Drawing for the job (mm, zero at the part's lowest x, y, z). A direction names the side the tool comes from. Coordinates: 2 decimals unless noted, no trailing zeros. Write each loop counter-clockwise with the first axis right and the second up, starting at its lowest first coordinate (ties: lowest second). Pieces come first, ordered by that corner, then holes.
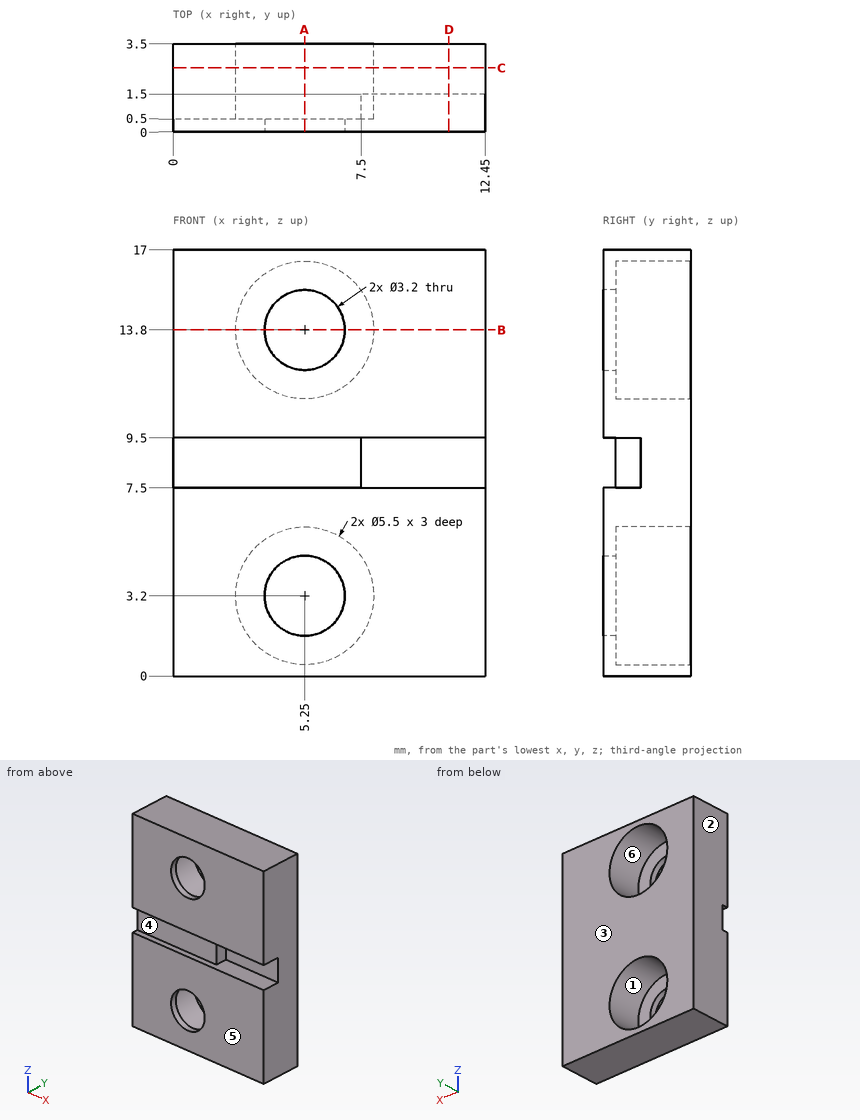
Item 1: Flat gauge pins, fed straight in: pin 1 Ø5 at (x, z) = (5.25, 3.2) entering from +Y; pin 2 Ø1.5 at (x, z) = (3, 13.5) entering from +Y; pin 3 Ø1.6 at (x, z) = (5, 8.5) entering from -Y. Where does each tip first touch, or does it go through?
Item 2: Two-plate mould, pull along X, no slides. Class the marked faces 1, 2 and 3: +X half, -X half, draft (parallel to the pull), parting line (faces both ways), or undercut.
Item 3: Wall check: line 1 along Z through (x, y) = (5.25, 0.15); line 2 along X through (y, z) = (2.8, 3.2); line 3 along Z through (x, y) = (8.75, 1.1). Give the ranges that are in metal, low to high.
Item 4: Which spindle directions (+Z, -Z, +X, -X, +Y, -Y) get a long thin tool onto all of the face, cutting with end or side? Do the marked faces 4, 5 and 6. Say none if no direction does.
Item 5: Saw through at A-A, the plane x = 5.25. Write the cut outline in (y, z), and give its area (3 significant figures).
Item 6: Saw through at B-B, the plane z = 13.8. Write the cut outline in (x, y), and give its area (3 significant figures).
Item 7: Saw through at C-C, the plane y = 2.55. Write the cut outline in (x, z).
Item 8: Saw through at D-D, the plane x = 11. Write the cut outline in (y, z).
Working result:
1. pin 1: stops at y = 0.5
1. pin 2: stops at y = 3.5
1. pin 3: stops at y = 0.5
2. face 1: undercut
2. face 2: -X half
2. face 3: draft
3. line 1: z = 0 to 1.6, 4.8 to 7.5, 9.5 to 12.2, 15.4 to 17
3. line 2: x = 0 to 2.5, 8 to 12.45
3. line 3: z = 0 to 7.5, 9.5 to 17
4. face 4: +X, -X, -Y
4. face 5: +Z, -Z, +X, -X, -Y
4. face 6: +Y
5. outline: (0, 0) - (3.5, 0) - (3.5, 0.45) - (0.5, 0.45) - (0.5, 1.6) - (0, 1.6) - close; (0, 4.8) - (0.5, 4.8) - (0.5, 5.95) - (3.5, 5.95) - (3.5, 11.05) - (0.5, 11.05) - (0.5, 12.2) - (0, 12.2) - (0, 9.5) - (0.5, 9.5) - (0.5, 7.5) - (0, 7.5) - close; (0, 15.4) - (0.5, 15.4) - (0.5, 16.55) - (3.5, 16.55) - (3.5, 17) - (0, 17) - close
5. area: 22.3 mm2
6. outline: (0, 0) - (3.65, 0) - (3.65, 0.5) - (2.5, 0.5) - (2.5, 3.5) - (0, 3.5) - close; (6.85, 0) - (12.45, 0) - (12.45, 3.5) - (8, 3.5) - (8, 0.5) - (6.85, 0.5) - close
6. area: 25.5 mm2
7. outline: (0, 0) - (12.45, 0) - (12.45, 17) - (0, 17) - close; hole circle Ø5.5 at (5.25, 3.2); hole circle Ø5.5 at (5.25, 13.8)
8. outline: (0, 0) - (3.5, 0) - (3.5, 17) - (0, 17) - (0, 9.5) - (1.5, 9.5) - (1.5, 7.5) - (0, 7.5) - close
